Part model, mm, in its own coordinate system. A direction names the side the tool comes from. Give positions to 0.01 mm unless a question says otherwise; leave off trailing zeros. Write each loop counter-clockwise with the first axis right and the second up, starting at its lowest first coordinate (ties: lowest second). Pieces come first, ordered by that corner, then holes.
from build123d import *

# Parameters (mm, degrees)
F1_DEPTH = 12.7
F2_DEPTH = 44.45
F3_W     = 31.75
F3_H     = 14.2875
F4_DEPTH = 44.45
F5_R     = 6.35
F6_DEPTH = 25.4


with BuildPart() as f1:
    # F0 (on Front) → F1 (new body)
    with BuildSketch(Plane.XZ):
        Polygon((30.037765, -41.944019), (61.787765, -41.944019), (61.787765, -19.719019), (14.162765, 27.905981), (-17.587235, 27.905981), (-65.212235, -19.719019), (-65.212235, -41.944019), (-33.462235, -41.944019), (-33.462235, -29.244019), (-14.412235, -10.194019), (-1.712235, -10.194019), (10.987765, -10.194019), (30.037765, -29.244019), align=None)
    extrude(amount=F1_DEPTH)

    # F0 (on Front) → F2 (join)
    with BuildSketch(Plane.XZ):
        Polygon((-33.462235, -41.944019), (30.037765, -41.944019), (30.037765, -29.244019), (10.987765, -10.194019), (-1.712235, -10.194019), (-14.412235, -10.194019), (-33.462235, -29.244019), align=None)
    extrude(amount=F2_DEPTH)

    # F3 (on face) → F4 (join)
    with BuildSketch(Plane.XZ.offset(12.7)):
        with Locations((-1.712235, 20.762231)):
            Rectangle(F3_W, F3_H)
    extrude(amount=F4_DEPTH)

    # F5 (on face) → F6 (cut)
    with BuildSketch(Plane.XY.offset(27.905981)):
        with Locations((-1.712235, -41.275)):
            Circle(F5_R)
    extrude(amount=-F6_DEPTH, mode=Mode.SUBTRACT)


solid = f1.part
1) 3-axis set-ups, long thin cutter, end or side, ignore diameter. For faces 1 (the flat face through (30.038, -28, -36)), 2 (the flat face through (-23.804, -28.353, -19.586)), 3 (the cylindrical face through (-3.089, -47.474, 20.862)), 4 (the flat face through (-1.9, -34.6, 13.618)), 5 (the flat face through (-33.462, -28, -36)): which of +Z, -Z, +X, -X, +Y, -Y reach the whole face in a straight line?
Check result:
face 1: +Z, -Z, +X, -Y
face 2: -X, -Y
face 3: +Z
face 4: +X, -X, -Y
face 5: +Z, -Z, -X, -Y
2) Saw through at A-A (y = -31.5). Write the cut outline in (x, z), and give its area (3 significant figures).
Check result:
outline: (-33.46, -41.94) - (30.04, -41.94) - (30.04, -29.24) - (10.99, -10.19) - (-14.41, -10.19) - (-33.46, -29.24) - close; (-17.59, 13.62) - (14.16, 13.62) - (14.16, 27.91) - (-17.59, 27.91) - close
area: 2,110 mm2
3) Flat gauge pins, fed straight in: P1, Ø14.5, axis at x = -1.71, y = -41.28, coming from the +Z side; P2, Ø10, axis at y = -26.5, z = -37.5, coming from the -X side; P3, Ø21, axis at x = -18, z = -13.5, coming from the -Y side; P4, Ø15.5, axis at y = -33, z = 19, coming from the +X side. Where does each tip first touch, or does it go through?
Check result:
P1: stops at z = 27.91
P2: stops at x = -33.46
P3: stops at y = -44.45
P4: stops at x = 14.16
4) Saw through at D-D (x = 17.5). Write the cut outline in (y, z), and give its area (3 significant figures).
Check result:
outline: (-44.45, -41.94) - (0, -41.94) - (0, 24.57) - (-12.7, 24.57) - (-12.7, -16.71) - (-44.45, -16.71) - close
area: 1,650 mm2
5) Saw through at C-C (z = -14.5). Write the cut outline in (x, y), and give its area (3 significant figures).
Check result:
outline: (-59.99, -12.7) - (-18.72, -12.7) - (-18.72, -44.45) - (15.29, -44.45) - (15.29, -12.7) - (56.57, -12.7) - (56.57, 0) - (-59.99, 0) - close
area: 2,560 mm2
6) Drill centre lines: L1, parallel to X at y = -41, z = -31; L2, parallel to Y at x = -33.5, z = -20; L3, parallel to Z at x = -7.5, y = -48. Where is each one in solid material? Low to high.
Check result:
L1: x = -33.46 to 30.04
L2: y = -12.7 to 0
L3: z = 13.62 to 27.91
7) Mould opens along Z. For faces 6 (the flat face through (-2, -28, -10.194)), 7 (the flat face through (14.163, -35, 21)), 8 (the flat face through (-2, -28, 27.906)) say: +Z half, -Z half, draft (parallel to the pull), parting line (faces both ways), or undercut.
Check result:
face 6: undercut
face 7: draft
face 8: +Z half
8) Saw through at B-B (z = 22). Write the cut outline in (x, y) (3 decimals), and give its area (3 significant figures).
Check result:
outline: (-23.493, -12.7) - (-17.587, -12.7) - (-17.587, -57.15) - (14.163, -57.15) - (14.163, -12.7) - (20.069, -12.7) - (20.069, 0) - (-23.493, 0) - close; hole circle Ø12.7 at (-1.712, -41.275)
area: 1,840 mm2
